Geometry check sheet. Reference: the model listing, model coordinates, mm. A direction names the side the tool comes from. Give positions to 0.01 mm unless a question says otherwise; leave off trailing zeros. Answer as a JSON object with one key per item and string values. Group by question number.
Autodesk Inventor part; units mm, degrees
ref_plane "YZ Plane" through (0, 0, 0) normal (1, 0, 0) x (0, 1, 0)
ref_plane "XZ Plane" through (0, 0, 0) normal (0, 1, 0) x (-1, 0, 0)
ref_plane "XY Plane" through (0, 0, 0) normal (0, 0, 1) x (1, 0, 0)
sketch "Skizze1" plane through (0, 0, 0) normal (1, 0, 0) x (0, 1, 0)
  line L0 (-125, 50) -> (125, 50)
  line L1 (125, 50) -> (125, -50)
  line L2 (125, -50) -> (-125, -50)
  line L3 (-125, -50) -> (-125, 50)
  line L4 (-125, 50) -> (125, -50) construction
  line L5 (125, 50) -> (-125, -50) construction
  point P0 (0, 0)
  dimension "d0" = 250
  dimension "d1" = 100
extrude "Extrusion1" add sketch "Skizze1" along normal blind 20
sketch "Skizze2" plane through (20, 0, 0) normal (1, 0, 0) x (0, 0, -1)
  line L0 (25, -23.5) -> (-25, -23.5)
  line L1 (-25, -23.5) -> (-25, -73.5)
  line L2 (-25, -73.5) -> (25, -73.5)
  line L3 (25, -73.5) -> (25, -23.5)
  line L4 (25, -23.5) -> (-25, -73.5) construction
  line L5 (-25, -23.5) -> (25, -73.5) construction
  line L6 (25, 73.5) -> (-25, 73.5)
  line L7 (-25, 73.5) -> (-25, 23.5)
  line L8 (-25, 23.5) -> (25, 23.5)
  line L9 (25, 23.5) -> (25, 73.5)
  line L10 (25, 73.5) -> (-25, 23.5) construction
  line L11 (-25, 73.5) -> (25, 23.5) construction
  point P0 (0, 0)
  point P1 (0, -48.5)
  point P2 (0, 48.5)
  point P3 (-19, -67.5)
  point P4 (-19, -29.5)
  point P5 (19, -29.5)
  point P6 (19, -67.5)
  point P7 (19, 29.5)
  point P8 (19, 67.5)
  point P9 (-19, 67.5)
  point P10 (-19, 29.5)
  dimension "d4" = 50
  dimension "d5" = 50
  dimension "d6" = 50
  dimension "d7" = 50
  dimension "d8" = 97
  dimension "d10" = 48.5
  dimension "d11" = 0
  dimension "d13" = 6
  dimension "d14" = 6
  dimension "d15" = 6
  dimension "d16" = 6
  dimension "d17" = 6
  dimension "d18" = 6
  dimension "d19" = 6
  dimension "d20" = 6
fillet "Rundung1" radius 10 4 edges at (10, -125, 50) (10, -125, -50) (10, 125, -50) (10, 125, 50)
hole "Bohrung1" at (20, -67.5, 19) at (20, -29.5, 19) at (20, -29.5, -19) at (20, -67.5, -19) at (20, 29.5, -19) at (20, 67.5, -19) at (20, 67.5, 19) at (20, 29.5, 19) direction (-1, 0, 0) diameter 4.134 depth 14.2
equation "\"d22\" = d19"
properties part number "Gehäuse festigung platte" material "Aluminium 6061"
1. Access from +Z, -Z, +X, -X, +Y, -Y to the whole of each face (thin tool, end or side, straight path). Record for faces 5 (the flat face through (5.8, 29, 19)), 6 (the cylindrical face through (10.14, -122.15, -46.99)).
2. Depth check by flat-ended pin: pin 1 (5.5 mm diameter, centred on y = 67.5, z = -19, fed in from -X); pin 2 (3.5 mm diameter, centred on y = -67.5, z = -19, fed in from +X). Enter the tip coordinate at first touch or a pass-through.
3. Release check for a two-part mould opening along Z. For faces 1 (the flat face through (10, -2, 50)), 2 (the flat face through (5.8, 67, 19)), 3 (the cylindrical face through (12.8, -68.12, 17.03)), 4 (the flat face through (0, -2, 1)) record: released by +Z, released by -Z, zero draft, split by the parting line, or undercut.
4. Thickness scan on line 1 along Y through (x, z) = (14.25, 19); line 2 along Z through (x, y) = (11.5, -67.5); line 3 along Y through (x, z) = (6, 46). Record the ranges inside material, lowest first. Write a range as [from, to].
Report:
{
 "1": {"face 5": "+X", "face 6": "-Z, +X, -X, -Y"},
 "2": {"pin 1": "stops at x = 0", "pin 2": "stops at x = 5.8"},
 "3": {"face 1": "released by +Z", "face 2": "undercut", "face 3": "undercut", "face 4": "zero draft"},
 "4": {"line 1": "y = [-125, -69.57], [-65.43, -31.57], [-27.43, 27.43], [31.57, 65.43], [69.57, 125]", "line 2": "z = [-50, -21.07], [-16.93, 16.93], [21.07, 50]", "line 3": "y = [-123, 123]"}
}
